```python
from build123d import *

# Parameters (mm, degrees)
CORTAR_EXTRUIR1_DEPTH = 22
CROQUIS5_OUTSIDE_W    = 102.148
CROQUIS5_OUTSIDE_H    = 102.148
CROQUIS5_OUTSIDE_R    = 1.5
CORTAR_EXTRUIR2_DEPTH = 5.5
CROQUIS6_R            = 1.5
CORTAR_EXTRUIR3_DEPTH = 10


with BuildPart() as part:
    # Croquis3 → Revolución1 (revolve)
    with BuildSketch(Plane.XY):
        with BuildLine():
            Line((-25.85, 65.019911999), (-18.85, 65.019911999))
            Line((-18.85, 65.019911999), (-18.85, 61.319911999))
            Line((-18.85, 61.319911999), (-4, 61.319911999))
            Line((-4, 61.319911999), (-4, 66.503346961))
            Line((-4, 66.503346961), (0, 66.503346961))
            Line((0, 66.503346961), (0, -136.580088001))
            Line((0, -136.580088001), (-9.6, -136.580088001))
            Line((-9.6, -136.580088001), (-9.6, -123.380088001))
            Line((-9.6, -123.380088001), (-6.9, -123.380088001))
            Line((-6.9, -123.380088001), (-6.9, -113.880088001))
            Line((-6.9, -113.880088001), (-8, -113.880088001))
            Line((-8, -113.880088001), (-8, -93.880088001))
            Line((-8, -93.880088001), (-4.75, -93.880088001))
            Line((-4.75, -93.880088001), (-4.75, -92.880088001))
            Line((-4.75, -92.880088001), (-13, -92.880088001))
            Line((-13, -92.880088001), (-13, -86.280088001))
            Line((-13, -86.280088001), (-22.9, -86.280088001))
            ThreePointArc((-22.9, -86.280088001), (-24.597056275, -85.577144276), (-25.3, -83.880088001))
            Line((-25.3, -83.880088001), (-25.3, -83.780088001))
            Line((-25.3, -83.780088001), (-26, -83.780088001))
            Line((-26, -83.780088001), (-26, 30.219911999))
            Line((-26, 30.219911999), (-25.3, 30.219911999))
            Line((-25.3, 30.219911999), (-25.3, 30.319911999))
            ThreePointArc((-25.3, 30.319911999), (-24.597056275, 32.016968273), (-22.9, 32.719911999))
            Line((-22.9, 32.719911999), (-13, 32.719911999))
            Line((-13, 32.719911999), (-13, 39.619911999))
            Line((-13, 39.619911999), (-28.25, 39.619911999))
            Line((-28.25, 39.619911999), (-28.25, 62.619911999))
            ThreePointArc((-28.25, 62.619911999), (-27.547056275, 64.316968273), (-25.85, 65.019911999))
        make_face()
    revolve(axis=Axis((0, 66.503346961, 0), (0, -1, 0)))

    # Croquis4 → Cortar-Extruir1 (cut)
    with BuildSketch(Plane(origin=(0, 61.319911999, 0), x_dir=(1, 0, 0), z_dir=(0, 1, 0))):
        with BuildLine():
            Line((-7.658154871, 1.479382123), (-18.690121594, 0.847087609))
            ThreePointArc((-18.690121594, 0.847087609), (-18.36871906, 4.212095184), (-17.32507143, 7.427274058))
            Line((-17.32507143, 7.427274058), (-7.454960737, 2.458873808))
            ThreePointArc((-7.454960737, 2.458873808), (-7.52975075, 2.219313777), (-7.596844825, 1.97748545))
            ThreePointArc((-7.596844825, 1.97748545), (-7.631481428, 1.728923867), (-7.658154871, 1.479382123))
        make_face()
        with BuildLine():
            Line((-5.64263548, 5.384846547), (-15.265160683, 10.817258061))
            ThreePointArc((-15.265160683, 10.817258061), (-13.175519219, 13.474319242), (-10.559290029, 15.614861321))
            Line((-10.559290029, 15.614861321), (-4.942144512, 6.098992345))
            ThreePointArc((-4.942144512, 6.098992345), (-5.134577805, 5.937896156), (-5.321763197, 5.770731017))
            ThreePointArc((-5.321763197, 5.770731017), (-5.485283899, 5.580353669), (-5.64263548, 5.384846547))
        make_face()
        with BuildLine():
            Line((-1.835619193, 7.58066024), (-6.993619113, 17.353025509))
            ThreePointArc((-6.993619113, 17.353025509), (-3.79918512, 18.458542146), (-0.441008652, 18.844840444))
            Line((-0.441008652, 18.844840444), (-0.860232323, 7.802723906))
            ThreePointArc((-0.860232323, 7.802723906), (-1.109212687, 7.771238461), (-1.357059356, 7.73181026))
            ThreePointArc((-1.357059356, 7.73181026), (-1.597547489, 7.660060609), (-1.835619193, 7.58066024))
        make_face()
        with BuildLine():
            Line((2.554193218, 7.369667869), (3.498347111, 18.379329969))
            ThreePointArc((3.498347111, 18.379329969), (6.78336341, 17.58230834), (9.817289856, 16.091715878))
            Line((9.817289856, 16.091715878), (3.49479755, 7.029145758))
            ThreePointArc((3.49479755, 7.029145758), (3.268319623, 7.137267463), (3.038501242, 7.238094376))
            ThreePointArc((3.038501242, 7.238094376), (2.79739896, 7.30775243), (2.554193218, 7.369667869))
        make_face()
        with BuildLine():
            Line((6.133067329, 4.818858021), (12.879612845, 13.570327026))
            ThreePointArc((12.879612845, 13.570327026), (15.212241987, 11.123815867), (16.9586682, 8.229585218))
            Line((16.9586682, 8.229585218), (6.740253894, 4.023863497))
            ThreePointArc((6.740253894, 4.023863497), (6.608183545, 4.237264476), (6.469359165, 4.44633467))
            ThreePointArc((6.469359165, 4.44633467), (6.304191006, 4.635284488), (6.133067329, 4.818858021))
        make_face()
        with BuildLine():
            Line((7.764735898, 0.7380948), (18.171692504, 4.452841136))
            ThreePointArc((18.171692504, 4.452841136), (18.811341218, 1.133590454), (18.715789216, -2.2453806))
            Line((18.715789216, -2.2453806), (7.845727251, -0.258966992))
            ThreePointArc((7.845727251, -0.258966992), (7.849995883, -0.008040044), (7.846241263, 0.242895122))
            ThreePointArc((7.846241263, 0.242895122), (7.80944695, 0.491146473), (7.764735898, 0.7380948))
        make_face()
        with BuildLine():
            Line((6.931155682, -3.577008305), (17.694388188, -6.078390353))
            ThreePointArc((17.694388188, -6.078390353), (16.437972526, -9.21654192), (14.530779394, -12.007453943))
            Line((14.530779394, -12.007453943), (6.460237641, -4.459577292))
            ThreePointArc((6.460237641, -4.459577292), (6.599489993, -4.250791906), (6.731997199, -4.037661911))
            ThreePointArc((6.731997199, -4.037661911), (6.835258667, -3.808927078), (6.931155682, -3.577008305))
        make_face()
        with BuildLine():
            Line((3.89698251, -6.756436547), (11.599240645, -14.679775853))
            ThreePointArc((11.599240645, -14.679775853), (8.845663703, -16.640487354), (5.732349785, -17.9572455))
            Line((5.732349785, -17.9572455), (3.023668226, -7.244303311))
            ThreePointArc((3.023668226, -7.244303311), (3.25369266, -7.143947373), (3.480391591, -7.036289816))
            ThreePointArc((3.480391591, -7.036289816), (3.690924052, -6.899693193), (3.89698251, -6.756436547))
        make_face()
        with BuildLine():
            Line((-0.374455074, -7.790743924), (1.821416153, -18.620436241))
            ThreePointArc((1.821416153, -18.620436241), (-1.555080846, -18.78119563), (-4.886060379, -18.20573849))
            Line((-4.886060379, -18.20573849), (-1.372894487, -7.729014215))
            ThreePointArc((-1.372894487, -7.729014215), (-1.125129102, -7.768950026), (-0.876213757, -7.80094542))
            ThreePointArc((-0.876213757, -7.80094542), (-0.62525287, -7.799855471), (-0.374455074, -7.790743924))
        make_face()
        with BuildLine():
            Line((-4.527005818, -6.351545152), (-8.534695097, -16.649239689))
            ThreePointArc((-8.534695097, -16.649239689), (-11.462098214, -14.959006995), (-13.953180895, -12.674038145))
            Line((-13.953180895, -12.674038145), (-5.3335729, -5.759817716))
            ThreePointArc((-5.3335729, -5.759817716), (-5.146730325, -5.927365938), (-4.954627427, -6.088855973))
            ThreePointArc((-4.954627427, -6.088855973), (-4.742916424, -6.223618748), (-4.527005818, -6.351545152))
        make_face()
        with BuildLine():
            Line((-7.242264201, -2.895775672), (-16.181100958, -9.392027173))
            ThreePointArc((-16.181100958, -9.392027173), (-17.729980386, -6.387439334), (-18.590265066, -3.11842024))
            Line((-18.590265066, -3.11842024), (-7.600879603, -1.961919789))
            ThreePointArc((-7.600879603, -1.961919789), (-7.534281034, -2.203885046), (-7.459981898, -2.443597775))
            ThreePointArc((-7.459981898, -2.443597775), (-7.354737525, -2.671427046), (-7.242264201, -2.895775672))
        make_face()
    extrude(amount=-CORTAR_EXTRUIR1_DEPTH, mode=Mode.SUBTRACT)

    # Croquis5 outside → Cortar-Extruir2 (cut)
    with BuildSketch(Plane.XZ.offset(136.580088001)):
        Rectangle(CROQUIS5_OUTSIDE_W, CROQUIS5_OUTSIDE_H)
        Polygon((9.814954576, 0), (4.907477288, 8.5), (-4.907477288, 8.5), (-9.814954576, 0), (-4.907477288, -8.5), (4.907477288, -8.5), align=None, mode=Mode.SUBTRACT)
        with Locations((-0.096894906, 0)):
            Circle(CROQUIS5_OUTSIDE_R)
    extrude(amount=-CORTAR_EXTRUIR2_DEPTH, mode=Mode.SUBTRACT)

    # Croquis6 → Cortar-Extruir3 (cut)
    with BuildSketch(Plane.XZ.offset(86.280088001)):
        with Locations((0, 17.5)):
            Circle(CROQUIS6_R)
        with Locations((17.5, 0)):
            Circle(CROQUIS6_R)
        with Locations((0, -17.5)):
            Circle(CROQUIS6_R)
        with Locations((-17.5, 0)):
            Circle(CROQUIS6_R)
    extrude(amount=-CORTAR_EXTRUIR3_DEPTH, mode=Mode.SUBTRACT)


solid = part.part
```
Verification items for the finished model (mm, model axes). A direction names the side the tool comes from. Coordinates: 2 decimals unless noted, no trailing zeros. Write each loop counter-clockwise with the first axis right and the second up, starting at its lowest first coordinate (ties: lowest second). Pieces come first, ordered by that corner, then holes. Notation, with made-up numbers: (18.5, 59.5) - (45.5, 59.5) arc R17 ccw to (45.5, 86.5) - close; hole circle Ø5 at (4, 70.5). An arc over 180 degrees is marked (long way). Write item = value, one per line.
Q1. Mould release check, pull along Y, two halves, no side actions. Record for faces 5 (the face through (-2.192, -93.373, 4.214)), 6 (the face through (0, -136.58, 2)), 7 (the face through (3.02, 50.47, -12.8)): released by +Y, released by -Y, zero draft, split by the parting line, or undercut.
Answer:
face_5 = undercut
face_6 = released by -Y
face_7 = zero draft
Q2. Access from +Z, -Z, +X, -X, +Y, -Y to the whole of each face (thin tool, end or side, straight path). Record for faces 1 (the face through (-7.33, -133.869, 4.304)), 2 (the face through (-7, 39.62, -13)), 3 (the face through (9.459, 50.474, -9.133)), 4 (the face through (-7.39, -133.87, -4.2)).
Answer:
face_1 = +Z, -X, -Y
face_2 = none
face_3 = +Y
face_4 = -Z, -X, -Y
Q3. Material ranges on L1, parallel to Z at x = 0, y = -79.5; L2, parallel to X at y = 63, z = 0; L3, parallel to Y at x = 1.5, z = -14.5, recorded low to high. Write a range as from..to.
Answer:
L1 = -26..-19, -16..16, 19..26
L2 = -28.22..-18.85, -4..4, 18.85..28.22
L3 = -86.28..32.72, 39.62..61.32
Q4. Cross-section at A-A (y = -55). Enter the section's corners in (x, z), plus the area to 3 significant figures.
Answer:
outline = circle Ø52 at (0, 0)
area = 2,120 mm²
Q5. Go/stop test with flat-tipped pins: pin 1 Ø2.5 at (x, z) = (-13, 13.5) entering from -Y; pin 2 Ø3 at (x, z) = (-9, 4) entering from +Y; pin 3 Ø12 at (y, z) = (-49, -3) entering from +X. Record where each tip stops, or that it passes through.
Answer:
pin_1 = -86.28
pin_2 = 61.32
pin_3 = 26
Q6. Cross-section at B-B (y = -97). Enter the section's corners in (x, z).
Answer:
outline = circle Ø16 at (0, 0)
